Autodesk Inventor part; units mm, degrees
ref_plane "Work Plane1" through (0, 28, 45) normal (0.7071, 0, -0.7071) x (0, 1, 0)
ref_plane "YZ Plane" through (0, 0, 0) normal (1, 0, 0) x (0, 1, 0)
ref_plane "XZ Plane" through (0, 0, 0) normal (0, 1, 0) x (-1, 0, 0)
sketch "Sketch1" plane through (0, 0, 0) normal (0, 0, 1) x (1, 0, 0)
  line L0 (0, 0) -> (138, 0)
  line L1 (138, 0) -> (138, 28)
  line L2 (138, 28) -> (0, 28)
  line L3 (0, 28) -> (0, 0)
  dimension "d0" = 138
  dimension "d1" = 28
extrude "Extrusion1" add sketch "Sketch1" along normal blind 45
ref_plane "Work Plane1" through (0, 28, 45) normal (0.7071, 0, -0.7071) x (0, 1, 0)
sketch "Sketch2" plane through (0, 28, 45) normal (0.7071, 0, -0.7071) x (0, 1, 0)
  line L0 (-28, 0) -> (0, 0)
  circle A0 centre (-3.049, 0) radius 1.5
  circle A1 centre (-5.7153, 0) radius 1.5
  circle A2 centre (-7.2153, 0.7211) radius 0.5
  circle A3 centre (-4.3663, 1.3485) radius 0.5
  circle A4 centre (-4.3663, -1.3706) radius 0.5
  point P0 (-28, -31.8198)
  dimension "d5" = 3
  dimension "d6" = 3
  dimension "d7" = 1
  dimension "d8" = 1
  dimension "d9" = 1
extrude "Extrusion2" add sketch "Sketch2" along normal mid plane 12.5 contours A1 A0 A3 L0 | A1 A0 L0 | L0 A0 A1 | L0 A0 A4 A1 | A0 A1 A4 L0 | L0 A1 A2 A3 A0 | A3 A0 | A0 A3 A1 | A4 A1 A0 | A0 A4 | A3 A1 | A1 A4 | A2 A1 | A1 A2 picked at (-4.3907, 1.3671) picked at (-4.3952, -1.3761)
fillet "Fillet1" radius 1 13 edges at (0, 10.3924, 45) (69, 28, 45) (69, 0, 45) (0, 27.2255, 45) (0, 28, 22.5) (0, 0, 22.5) (0, 14, 0) (69, 28, 0) (138, 28, 22.5) (138, 14, 45) (138, 0, 22.5) (138, 14, 0) (69, 0, 0)
properties part number "LiPoBattery"
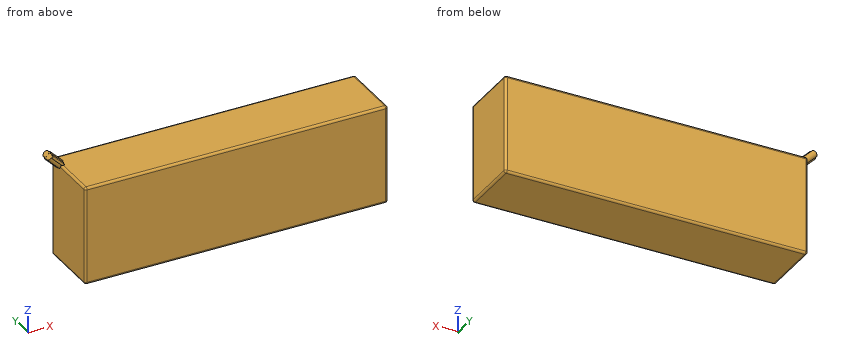
The listing builds one solid part. Answer for the finished solid, in the listing's coordinates (mm). Give positions to 0.01 mm unless a question says otherwise; leave off trailing zeros. Write each loop counter-clockwise with the first axis right and the second up, starting at its lowest first coordinate (ties: lowest second). Pieces come first, ordered by that corner, then holes.
1) Given P1, Ø2, axis at y = 5.5, z = 17.5, coming from the -X side; P2, Ø1.5, axis at x = 86.5, y = 8.5, coming from the +Z side, each flat-ended and moving along its own axis, determine where each tip first touches the part or whether it passes through.
2) Find the intervals of material crossed by L1, parallel to Z at x = 34.5, y = 7.5; L2, parallel to X at y = 6.5, z = 14, in increasing order.
3) Section A-A (y = 17) is taken. Write down the section's boundary in (x, z).
4) Section B-B (z = 29.5) is taken. Write down the section's boundary in (x, y).
Response:
1. P1: stops at x = 0
1. P2: stops at z = 45
2. L1: z = 0 to 45
2. L2: x = 0 to 138
3. outline: (0, 1) arc R1 ccw to (1, 0) - (137, 0) arc R1 ccw to (138, 1) - (138, 44) arc R1 ccw to (137, 45) - (1, 45) arc R1 ccw to (0, 44) - close
4. outline: (0, 1) arc R1 ccw to (1, 0) - (137, 0) arc R1 ccw to (138, 1) - (138, 27) arc R1 ccw to (137, 28) - (1, 28) arc R1 ccw to (0, 27) - close
